from build123d import *

# Parameters (mm, degrees)
SALIENTE_EXTRUIR1_DEPTH    = 10
CROQUIS2_R                 = 3.3
CORTAR_EXTRUIR1_DEPTH      = 29.495613698
CORTAR_EXTRUIR2_DEPTH      = 29.495613698
CORTAR_EXTRUIR2_DEPTH_BACK = 29.495613698
CROQUIS3_R                 = 1.5
CROQUIS4_R                 = 3.25
CORTAR_EXTRUIR3_DEPTH      = 1


with BuildPart() as part:
    # Croquis1 → Saliente-Extruir1 (new body)
    with BuildSketch(Plane(origin=(0, 0, 0), x_dir=(1, 0, 0), z_dir=(0, 1, 0))):
        with BuildLine():
            Line((-20, 6), (20, 6))
            ThreePointArc((20, 6), (26, 0), (20, -6))
            Line((20, -6), (-20, -6))
            ThreePointArc((-20, -6), (-26, 0), (-20, 6))
        make_face()
    extrude(amount=SALIENTE_EXTRUIR1_DEPTH)

    # Croquis2 → Cortar-Extruir1 (cut, through all)
    with BuildSketch(Plane(origin=(0, 0, 0), x_dir=(1, 0, 0), z_dir=(0, 1, 0))):
        with Locations(Location((-20, 0, 0), (0, 0, 270))):
            Circle(CROQUIS2_R)
        with Locations(Location((20, 0, 0), (0, 0, 270))):
            Circle(CROQUIS2_R)
    extrude(amount=CORTAR_EXTRUIR1_DEPTH, mode=Mode.SUBTRACT)

    # Croquis3 → Cortar-Extruir2 (cut, two sides: drawn at the far end of the back side and taken through both)
    with BuildSketch(Plane.XY.offset(-CORTAR_EXTRUIR2_DEPTH_BACK)):
        with Locations(Location((-20, 5, 0), (0, 0, 89.999999997))):
            Circle(CROQUIS3_R)
        with Locations(Location((20, 5, 0), (0, 0, 89.999999997))):
            Circle(CROQUIS3_R)
    extrude(amount=CORTAR_EXTRUIR2_DEPTH + CORTAR_EXTRUIR2_DEPTH_BACK, mode=Mode.SUBTRACT)

    # Croquis4 → Cortar-Extruir3 (cut)
    with BuildSketch(Plane.XY.offset(6)):
        with Locations((-20, 5)):
            Circle(CROQUIS4_R)
        with Locations(Location((20, 5, 0), (0, 0, 270.000000001))):
            Circle(CROQUIS4_R)
    extrude(amount=-CORTAR_EXTRUIR3_DEPTH, mode=Mode.SUBTRACT)


solid = part.part
Could you check a few things on this model? Use its own coordinates, in mm. A direction names the side the tool comes from. Give positions to 0.01 mm unless a question says otherwise; leave off trailing zeros. Order: outer loops, then holes, each group sorted by start corner. A loop starts at its lowest first (then second) coordinate and runs counter-clockwise, first axis right, second up.
Item 1: If we section it at D-D, the plane z = -5: Write out the boundary of the cut face in (x, y).
Item 2: If we mould it in two halves opening along Y, with no side actions, what happens to faces 3 (the face through (0, 5, 6)), 4 (the face through (19.3, 6.5, 5)), 5 (the face through (0, 10, 0))? For each: pulls with the +Y half, pulls with the -Y half, needs draft (parallel to the pull), parting line crosses it, or undercut.
Item 3: For faces 1 (the face through (-16.9, 5.98, 5.51)), 2 (the face through (18.513, 4.805, -4.491)), which set-ups out of +Z, -Z, +X, -X, +Y, -Y let a thin tool reach every point of the face, with its end or its side?
Item 4: If we section it at B-B, the plane z = -1.5: Write out the boundary of the cut face in (x, y).
Item 5: I need wall thicknesses on line 1 (X direction, y = 1.75, z = 0); line 2 (X direction, y = 6.25, z = 3.5); line 3 (Z direction, x = 20, y = 3.25). Which ranges of each line are inside material? Lowest first, please.
Item 6: If we section it at A-A, the plane y = 5: Write out the boundary of the cut face in (x, z).
Item 7: I'm going to push flat-ended pins straight in: pin 1 (5 mm diameter, centred on x = -20, y = 4.5, fed in from +Z); pin 2 (2.5 mm diameter, centred on x = 20, y = 5, fed in from -Z); pin 3 (2 mm diameter, centred on y = 8, z = -0.5, fed in from +X). Where does each tip first touch, or does it pass through?
Item 8: If we section it at C-C, the plane y = 7: Write out the boundary of the cut face in (x, z), plus the area to 3 significant figures.
Values:
1. outline: (-23.32, 0) - (23.32, 0) - (23.32, 10) - (-23.32, 10) - close; hole circle Ø3 at (-20, 5); hole circle Ø3 at (20, 5)
2. face 3: needs draft
2. face 4: undercut
2. face 5: pulls with the +Y half
3. face 1: +Z
3. face 2: +Z, -Z
4. outline: (-25.81, 0) - (-22.94, 0) - (-22.94, 10) - (-25.81, 10) - close; (-17.06, 0) - (17.06, 0) - (17.06, 10) - (-17.06, 10) - close; (22.94, 0) - (25.81, 0) - (25.81, 10) - (22.94, 10) - close
5. line 1: x = -26 to -23.3, -16.7 to 16.7, 23.3 to 26
5. line 2: x = -24.87 to -20.83, -19.17 to 19.17, 20.83 to 24.87
5. line 3: z = -6 to -3.3, 3.3 to 5
6. outline: (-23.25, 5) - (-23.25, 5.04) arc R6 ccw to (-21.5, -5.81) - (-21.5, -2.94) arc R3.3 cw to (-21.5, 2.94) - (-21.5, 5) - close; (-18.5, -6) - (18.5, -6) - (18.5, -2.94) arc R3.3 cw to (18.5, 2.94) - (18.5, 5) - (16.75, 5) - (16.75, 6) - (-16.75, 6) - (-16.75, 5) - (-18.5, 5) - (-18.5, 2.94) arc R3.3 cw to (-18.5, -2.94) - close; (21.5, -5.81) arc R6 ccw to (23.25, 5.04) - (23.25, 5) - (21.5, 5) - (21.5, 2.94) arc R3.3 cw to (21.5, -2.94) - close
7. pin 1: stops at z = 5
7. pin 2: passes through
7. pin 3: stops at x = 26
8. outline: (-22.56, 5) - (-22.56, 5.43) arc R6 ccw to (-20, -6) - (20, -6) arc R6 ccw to (22.56, 5.43) - (22.56, 5) - (17.44, 5) - (17.44, 6) - (-17.44, 6) - (-17.44, 5) - close; hole circle Ø6.6 at (-20, 0); hole circle Ø6.6 at (20, 0)
8. area: 515 mm2
